```python
from build123d import *

# Parameters (mm, degrees)
SALIENTE_EXTRUIR1_START      = 9
CROQUIS1_R                   = 6
CROQUIS1_R_2                 = 5.2
SALIENTE_EXTRUIR1_DEPTH      = 3
SALIENTE_EXTRUIR2_START      = 9
CROQUIS1_3_R                 = 6
SALIENTE_EXTRUIR2_DEPTH      = 4
SALIENTE_EXTRUIR3_START      = -9
CROQUIS1_4_R                 = 7
CROQUIS1_4_R_2               = 6
SALIENTE_EXTRUIR3_DEPTH      = 4
SALIENTE_EXTRUIR4_START      = -9
CROQUIS1_5_R                 = 6
CROQUIS1_5_R_2               = 5.2
SALIENTE_EXTRUIR4_DEPTH      = 3
SALIENTE_EXTRUIR5_DEPTH      = 7
SALIENTE_EXTRUIR5_DEPTH_BACK = 7
CROQUIS3_R                   = 1.7
CORTAR_EXTRUIR1_DEPTH        = 7
CROQUIS4_R                   = 1.7
CORTAR_EXTRUIR2_DEPTH        = 7
CROQUIS5_R                   = 3.2
CORTAR_EXTRUIR3_DEPTH        = 3.4
CROQUIS6_R                   = 3.2
CORTAR_EXTRUIR4_DEPTH        = 3.4
REDONDEO1_R                  = 8
SALIENTE_EXTRUIR6_START      = 9
SALIENTE_EXTRUIR6_DEPTH      = 4
SALIENTE_EXTRUIR7_DEPTH      = 13


with BuildPart() as part:
    # Croquis1 → Saliente-Extruir1 (new body)
    with BuildSketch(Plane(origin=(0, 0, 0), x_dir=(0, 0, -1), z_dir=(1, 0, 0)).offset(SALIENTE_EXTRUIR1_START)):
        Circle(CROQUIS1_R)
        Circle(CROQUIS1_R_2, mode=Mode.SUBTRACT)
    extrude(amount=-SALIENTE_EXTRUIR1_DEPTH)

    # Croquis1<3> → Saliente-Extruir2 (add)
    with BuildSketch(Plane(origin=(0, 0, 0), x_dir=(0, 0, -1), z_dir=(1, 0, 0)).offset(SALIENTE_EXTRUIR2_START)):
        with BuildLine():
            Line((-7, 7), (-7, 0))
            ThreePointArc((-7, 0), (0, -7), (7, 0))
            Line((7, 0), (7, 7))
            Line((7, 7), (-7, 7))
        make_face()
        Circle(CROQUIS1_3_R, mode=Mode.SUBTRACT)
    extrude(amount=-SALIENTE_EXTRUIR2_DEPTH)



with BuildPart() as body_2:
    # Croquis1<4> → Saliente-Extruir3 (new body)
    with BuildSketch(Plane(origin=(0, 0, 0), x_dir=(0, 0, -1), z_dir=(1, 0, 0)).offset(SALIENTE_EXTRUIR3_START)):
        with BuildLine():
            Line((-7, 7), (-7, 0))
            ThreePointArc((-7, 0), (-4.949747468, 4.949747468), (0, 7))
            Line((0, 7), (-7, 7))
        make_face()
        with BuildLine():
            ThreePointArc((0, 7), (4.949747468, 4.949747468), (7, 0))
            Line((7, 0), (7, 7))
            Line((7, 7), (0, 7))
        make_face()
        Circle(CROQUIS1_4_R)
        Circle(CROQUIS1_4_R_2, mode=Mode.SUBTRACT)
    extrude(amount=SALIENTE_EXTRUIR3_DEPTH)

    # Croquis1<5> → Saliente-Extruir4 (add)
    with BuildSketch(Plane(origin=(0, 0, 0), x_dir=(0, 0, -1), z_dir=(1, 0, 0)).offset(SALIENTE_EXTRUIR4_START)):
        Circle(CROQUIS1_5_R)
        Circle(CROQUIS1_5_R_2, mode=Mode.SUBTRACT)
    extrude(amount=SALIENTE_EXTRUIR4_DEPTH)


with BuildPart() as part_1:
    add(part.part)

    add(body_2.part)  # Saliente-Extruir5 merges body 2
    # Croquis2 → Saliente-Extruir5 (add, two sides)
    with BuildSketch(Plane.XY) as saliente_extruir5_sk:
        Polygon((9, 16), (17.960512242, 24.960512242), (17.960512242, 34.860007179), (0, 16.899494937), (-17.960512242, 34.860007179), (-17.960512242, 24.960512242), (-9, 16), (-9, 7), (9, 7), align=None)
    extrude(amount=SALIENTE_EXTRUIR5_DEPTH)
    extrude(saliente_extruir5_sk.sketch, amount=-SALIENTE_EXTRUIR5_DEPTH_BACK)

    # Croquis3 → Cortar-Extruir1 (cut)
    with BuildSketch(Plane(origin=(8.449747468, 8.449747468, 0), x_dir=(0.7071067811865509, -0.7071067811865441, 0), z_dir=(0.7071067811865441, 0.7071067811865509, 0))):
        with Locations(Location((-24.649747468, 0, 0), (0, 0, 180))):
            Circle(CROQUIS3_R)
    extrude(amount=-CORTAR_EXTRUIR1_DEPTH, mode=Mode.SUBTRACT)

    # Croquis4 → Cortar-Extruir2 (cut)
    with BuildSketch(Plane(origin=(-8.449747468, 8.449747468, 0), x_dir=(0.7071067811865509, 0.7071067811865441, 0), z_dir=(-0.7071067811865441, 0.7071067811865509, 0))):
        with Locations(Location((24.649747468, 0, 0), (0, 0, 180))):
            Circle(CROQUIS4_R)
    extrude(amount=-CORTAR_EXTRUIR2_DEPTH, mode=Mode.SUBTRACT)

    # Croquis5 → Cortar-Extruir3 (cut)
    with BuildSketch(Plane(origin=(-3.5, 3.5, 0), x_dir=(-0.7071067811865511, -0.707106781186544, 0), z_dir=(0.707106781186544, -0.7071067811865511, 0))):
        with Locations(Location((-24.649747468, 0, 0), (0, 0, 180))):
            Circle(CROQUIS5_R)
    extrude(amount=-CORTAR_EXTRUIR3_DEPTH, mode=Mode.SUBTRACT)

    # Croquis6 → Cortar-Extruir4 (cut)
    with BuildSketch(Plane(origin=(3.5, 3.5, 0), x_dir=(-0.7071067811865512, 0.7071067811865438, 0), z_dir=(-0.7071067811865438, -0.7071067811865512, 0))):
        with Locations(Location((24.649747468, 0, 0), (0, 0, 180))):
            Circle(CROQUIS6_R)
    extrude(amount=-CORTAR_EXTRUIR4_DEPTH, mode=Mode.SUBTRACT)

    # Redondeo1
    redondeo1_edges = [part_1.edges().sort_by_distance(p)[0] for p in [
        (9, 16, 0),
        (-9, 16, 0),
    ]]
    fillet(redondeo1_edges, radius=REDONDEO1_R)



with BuildPart() as body_2_2:
    # Croquis7 → Saliente-Extruir6 (new body)
    with BuildSketch(Plane.XY.offset(7).offset(SALIENTE_EXTRUIR6_START)):
        with BuildLine():
            Line((-17.960512242, 34.860007179), (0, 16.899494937))
            Line((0, 16.899494937), (17.960512242, 34.860007179))
            Line((17.960512242, 34.860007179), (12.785288814, 85.146653693))
            ThreePointArc((12.785288814, 85.146653693), (12.796319785, 85.003519062), (12.8, 84.860007179))
            Line((12.8, 84.860007179), (12.8, 34.860007179))
            ThreePointArc((12.8, 34.860007179), (10, 32.060007179), (7.2, 34.860007179))
            ThreePointArc((7.2, 34.860007179), (0, 27.660007179), (-7.2, 34.860007179))
            ThreePointArc((-7.2, 34.860007179), (-10, 32.060007179), (-12.8, 34.860007179))
            Line((-12.8, 34.860007179), (-12.8, 84.860007179))
            ThreePointArc((-12.8, 84.860007179), (-12.796319785, 85.003519062), (-12.785288814, 85.146653693))
            Line((-12.785288814, 85.146653693), (-17.960512242, 34.860007179))
        make_face()
        with BuildLine():
            ThreePointArc((-12.8, 84.860007179), (-10, 87.660007179), (-7.2, 84.860007179))
            Line((-7.2, 84.860007179), (-7.2, 34.860007179))
            ThreePointArc((-7.2, 34.860007179), (-10, 32.060007179), (-12.8, 34.860007179))
            Line((-12.8, 34.860007179), (-12.8, 84.860007179))
        make_face()
        with BuildLine():
            Line((-11.5, 84.860007179), (-11.5, 34.860007179))
            ThreePointArc((-11.5, 34.860007179), (-10, 33.360007179), (-8.5, 34.860007179))
            Line((-8.5, 34.860007179), (-8.5, 84.860007179))
            ThreePointArc((-8.5, 84.860007179), (-10, 86.360007179), (-11.5, 84.860007179))
        make_face(mode=Mode.SUBTRACT)
        with BuildLine():
            Line((12.8, 84.860007179), (12.8, 34.860007179))
            ThreePointArc((12.8, 34.860007179), (10, 32.060007179), (7.2, 34.860007179))
            Line((7.2, 34.860007179), (7.2, 84.860007179))
            ThreePointArc((7.2, 84.860007179), (10, 87.660007179), (12.8, 84.860007179))
        make_face()
        with BuildLine():
            ThreePointArc((11.5, 84.860007179), (10, 86.360007179), (8.5, 84.860007179))
            Line((8.5, 84.860007179), (8.5, 34.860007179))
            ThreePointArc((8.5, 34.860007179), (10, 33.360007179), (11.5, 34.860007179))
            Line((11.5, 34.860007179), (11.5, 84.860007179))
        make_face(mode=Mode.SUBTRACT)
        with BuildLine():
            Line((0, 87.660007179), (-10, 87.660007179))
            ThreePointArc((-10, 87.660007179), (-8.020101013, 86.839906166), (-7.2, 84.860007179))
            Line((-7.2, 84.860007179), (0, 84.860007179))
            Line((0, 84.860007179), (0, 87.660007179))
        make_face()
        with BuildLine():
            ThreePointArc((7.2, 84.860007179), (8.020101013, 86.839906166), (10, 87.660007179))
            Line((10, 87.660007179), (0, 87.660007179))
            Line((0, 87.660007179), (0, 84.860007179))
            Line((0, 84.860007179), (7.2, 84.860007179))
        make_face()
    extrude(amount=SALIENTE_EXTRUIR6_DEPTH)


with BuildPart() as part_2:
    add(part_1.part)

    add(body_2_2.part)  # Saliente-Extruir7 merges body 2 2
    # Croquis7<4> → Saliente-Extruir7 (add)
    with BuildSketch(Plane.XY.offset(7)):
        with BuildLine():
            ThreePointArc((-9, 12.686291501), (-9.60896374, 15.74775896), (-11.343145751, 18.343145751))
            Line((-11.343145751, 18.343145751), (-17.960512242, 24.960512242))
            Line((-17.960512242, 24.960512242), (-17.960512242, 34.860007179))
            Line((-17.960512242, 34.860007179), (0, 16.899494937))
            Line((0, 16.899494937), (17.960512242, 34.860007179))
            Line((17.960512242, 34.860007179), (17.960512242, 24.960512242))
            Line((17.960512242, 24.960512242), (11.343145751, 18.343145751))
            ThreePointArc((11.343145751, 18.343145751), (9.60896374, 15.74775896), (9, 12.686291501))
            Line((9, 12.686291501), (-9, 12.686291501))
        make_face()
    extrude(amount=SALIENTE_EXTRUIR7_DEPTH)


solid = part_2.part
```
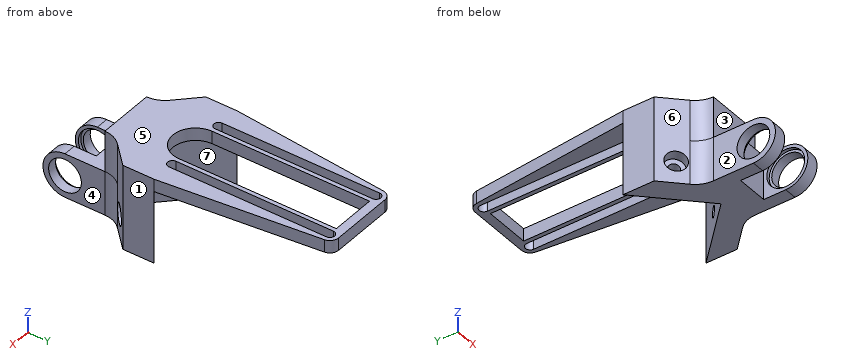
The listing builds one solid part. Answer for the finished solid, in the listing's coordinates (mm). Face numbers are marked on the shaded views. A direction names the side the tool comes from. Give positions to 0.01 mm unless a question says otherwise; leave off trailing zeros. Order: outer loops, then holes, each group sorted by start corner. A loop starts at its lowest first (then second) coordinate and runs counter-clockwise, first axis right, second up. Notation, with made-up numbers: (34.25, -13.75) - (74.25, -13.75) arc R30 cw to (74.25, 19.25) - close; hole circle Ø6 at (3, 38). An arc over 180 degrees is marked (long way). Use one line per item in the form item = value. Start each with the question number.
(1) For the marked faces 1, 2 and 3, determine the directions among +Z, -Z, +X, -X, +Y, -Y from which every point of the face is accessible in a straight line to the end or side of a thin tool.
(2) The mould has two halves that part along X. Classify the marked faces 4, 5, 6 and 7: released by +X, released by -X, zero draft, split by the parting line, or undercut.
(3) A cutting plane is placed at B-B, the plane z = 18.25. Write down the section's boundary in (x, y), then the cut area to 3 significant figures.
(4) A cutting plane is placed at C-C, the plane z = 8. Write down the section's boundary in (x, y), then the cut area to 3 significant figures.
(5) A cutting plane is placed at D-D, the plane z = 0. State how many separate pieces and enclosed holes the cut face has, then the cut area to 3 significant figures.
(6) Flat-ended cylindrical pins translate along their axes: pin 1 Ø8 at (x, z) = (-13.5, 6) entering from +Y; pin 2 Ø10 at (x, y) = (4.5, 6) entering from +Z; pin 3 Ø8 at (y, z) = (12, -1) entering from -X. Find the tip coordinate at first contact, or state that the pin passes through.
(7) Consider line 1 (Z direction, x = -12.5, y = 57); line 2 (Y direction, x = -7.65, z = 0); line 3 (Y direction, x = 8.2, z = 0). Determine where each line is inside the solid, lowest interval first. Write a range as from..to.
(8) A cutting plane is placed at A-A, the plane y = 49. Write down the section's boundary in (x, z), then the cut area to 3 significant figures.
Ans:
q1.face_1 = +Z, -Z, +X, +Y, -Y
q1.face_2 = +Z, -Z, -X, -Y
q1.face_3 = +Z, +X, -X, -Y
q2.face_4 = released by +X
q2.face_5 = zero draft
q2.face_6 = released by -X
q2.face_7 = undercut
q3.outline = (-17.96, 24.96) - (-11.34, 18.34) arc R8 cw to (-9, 12.69) - (9, 12.69) arc R8 cw to (11.34, 18.34) - (17.96, 24.96) - (17.96, 34.86) - (12.79, 85.15) arc R2.8 ccw to (10, 87.66) - (-10, 87.66) arc R2.8 ccw to (-12.79, 85.15) - (-17.96, 34.86) - close; hole (-11.5, 34.86) arc R1.5 ccw to (-8.5, 34.86) - (-8.5, 84.86) arc R1.5 ccw to (-11.5, 84.86) - close; hole (-7.2, 34.86) arc R7.2 ccw to (7.2, 34.86) - (7.2, 84.86) - (-7.2, 84.86) - close; hole (8.5, 34.86) arc R1.5 ccw to (11.5, 34.86) - (11.5, 84.86) arc R1.5 ccw to (8.5, 84.86) - close
q3.area = 1,150 mm^2
q4.outline = (-17.96, 24.96) - (-11.34, 18.34) arc R8 cw to (-9, 12.69) - (9, 12.69) arc R8 cw to (11.34, 18.34) - (17.96, 24.96) - (17.96, 34.86) - (0, 16.9) - (-17.96, 34.86) - close
q4.area = 337 mm^2
q5.separate_pieces = 5
q5.enclosed_holes = 0
q5.area = 397 mm^2
q6.pin_1 = 34.4
q6.pin_2 = 7
q6.pin_3 = -9.72
q7.line_1 = 16..20
q7.line_2 = -7..-5.2, 5.2..24.55
q7.line_3 = -7..-5.2, 5.2..24.26
q8.outline = (-16.51, 16) - (-11.5, 16) - (-11.5, 20) - (-16.51, 20) - close; (-8.5, 16) - (-7.2, 16) - (-7.2, 20) - (-8.5, 20) - close; (7.2, 16) - (8.5, 16) - (8.5, 20) - (7.2, 20) - close; (11.5, 16) - (16.51, 16) - (16.51, 20) - (11.5, 20) - close
q8.area = 50.4 mm^2
